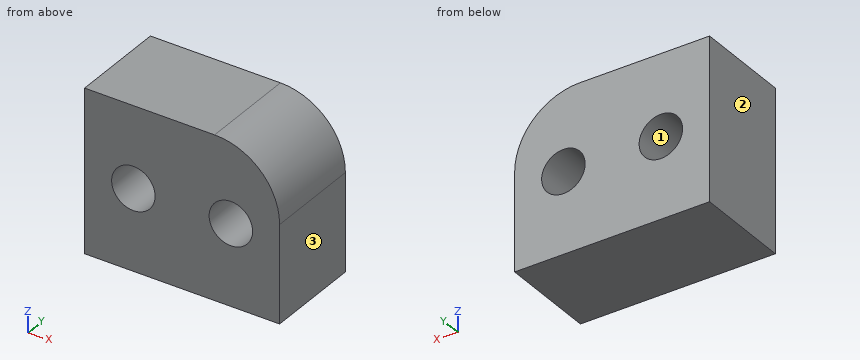
from build123d import *

# Parameters (mm, degrees)
SKETCH1_W           = 15.24
SKETCH1_H           = 12.7
SKETCH1_R           = 1.7
BOSS_EXTRUDE1_DEPTH = 7.62
FILLET1_R           = 5.08


with BuildPart() as part:
    # Sketch1 → Boss-Extrude1 (new body)
    with BuildSketch(Plane(origin=(0, 0, 0), x_dir=(1, 0, 0), z_dir=(0, 1, 0))):
        with Locations((7.62, 6.35)):
            Rectangle(SKETCH1_W, SKETCH1_H)
        with Locations(Location((11.43, 6.35, 0), (0, 0, 90))):
            Circle(SKETCH1_R, mode=Mode.SUBTRACT)
        with Locations(Location((3.81, 6.35, 0), (0, 0, 90))):
            Circle(SKETCH1_R, mode=Mode.SUBTRACT)
    extrude(amount=BOSS_EXTRUDE1_DEPTH)

    # Fillet1
    fillet1_edges = [part.edges().sort_by_distance(p)[0] for p in [
        (15.24, 3.81, 0),
    ]]
    fillet(fillet1_edges, radius=FILLET1_R)


solid = part.part
The model under review builds one solid part; all positions refer to its coordinate system, in mm. Face numbers are marked on the shaded views. Coordinates: 2 decimals unless noted, no trailing zeros. Write each loop counter-clockwise with the first axis right and the second up, starting at its lowest first coordinate (ties: lowest second). Pieces come first, ordered by that corner, then holes. Notation, with made-up numbers: (26, -32.75) -> (53, -32.75) arc R26 cw to (53, 3.25) -> close; hole circle Ø9 at (17.25, -15). An arc over 180 degrees is marked (long way). Answer in a Markdown table with one row per item.
1. Draft analysis for pull direction X (two halves, no side actions). For the marked faces 1, 2 and 3, state which applies: +X half, -X half, draft (parallel to the pull), parting line (faces both ways), or undercut.
Answers below:
| item | result |
|---|---|
| face 1 | undercut |
| face 2 | -X half |
| face 3 | +X half |
2. We need section A-A, the plane z = -6.35. State the section outline as (x, y) points, and give its area (3 significant figures).
Answers below:
| item | result |
|---|---|
| outline | (0, 0) -> (2.11, 0) -> (2.11, 7.62) -> (0, 7.62) -> close; (5.51, 0) -> (9.73, 0) -> (9.73, 7.62) -> (5.51, 7.62) -> close; (13.13, 0) -> (15.24, 0) -> (15.24, 7.62) -> (13.13, 7.62) -> close |
| area | 64.3 mm^2 |
3. We need section D-D, the plane x = 11.25. State the section outline as (y, z) points, and give its area (3 significant figures).
Answers below:
| item | result |
|---|---|
| outline | (0, -12.7) -> (7.62, -12.7) -> (7.62, -8.04) -> (0, -8.04) -> close; (0, -4.66) -> (7.62, -4.66) -> (7.62, -0.12) -> (0, -0.12) -> close |
| area | 70.1 mm^2 |
4. Wall thickness on probe 1 along X at (y, z) = (4.5, -6.35); probe 2 along X at (y, z) = (3, -5); probe 3 along Z at (x, y) = (3, 4.75): over which ranges is each line inside the solid? List them lowest first. Write a range as [from, to].
Answers below:
| item | result |
|---|---|
| probe 1 | x = [0, 2.11], [5.51, 9.73], [13.13, 15.24] |
| probe 2 | x = [0, 2.78], [4.84, 10.4], [12.46, 15.24] |
| probe 3 | z = [-12.7, -7.84], [-4.86, 0] |
5. We need section B-B, the plane x = 3.81. State the section outline as (y, z) points, and give its area (3 significant figures).
Answers below:
| item | result |
|---|---|
| outline | (0, -12.7) -> (7.62, -12.7) -> (7.62, -8.05) -> (0, -8.05) -> close; (0, -4.65) -> (7.62, -4.65) -> (7.62, 0) -> (0, 0) -> close |
| area | 70.9 mm^2 |
6. We need section C-C, the plane y = 1.25. State the section outline as (x, z) points, and give its area (3 significant figures).
Answers below:
| item | result |
|---|---|
| outline | (0, -12.7) -> (15.24, -12.7) -> (15.24, -5.08) arc R5.08 ccw to (10.16, 0) -> (0, 0) -> close; hole circle Ø3.4 at (3.81, -6.35); hole circle Ø3.4 at (11.43, -6.35) |
| area | 170 mm^2 |
7. Clearance check with a flat-ended pin moving along its axis: pin 1 Ø4 at (x, z) = (11.43, -6.35) entering from +Y. State where the tip first meets the part, or that it passes through.
Answers below:
| item | result |
|---|---|
| pin 1 | stops at y = 7.62 |
